Input: part model. Units: mm. Frame: model coordinates. Face numbers are marked on the shaded views. Give positions to 0.01 mm unless a question says otherwise; leave off trailing zeros. Write each loop counter-clockwise with the first axis right and the second up, starting at its lowest first coordinate (ties: lowest second). Pieces come first, ordered by that corner, then holes. Notation, with made-up numbers: (-6, 19) -> (3, 19) arc R27 cw to (3, 54) -> close; hole circle Ø8 at (12, 49.5). An arc over 180 degrees is marked (long way). Answer as a JSON object with one key per item and string values. Group by question number.
Autodesk Inventor part; units mm, degrees
ref_plane "YZ Plane" through (0, 0, 0) normal (1, 0, 0) x (0, 1, 0)
ref_plane "XZ Plane" through (0, 0, 0) normal (0, 1, 0) x (-1, 0, 0)
ref_plane "XY Plane" through (0, 0, 0) normal (0, 0, 1) x (1, 0, 0)
sketch "Sketch_1" plane through (0, 0, 0) normal (0, 0, 1) x (1, 0, 0)
  line L0 (12, 0) -> (-0.8, 0)
  line L1 (-0.8, 0) -> (-0.8, 2)
  line L2 (-0.8, 2) -> (-0.2226, 3)
  line L3 (-0.2226, 3) -> (0, 3)
  line L4 (0, 3) -> (0, 1.4467)
  arc A0 (0, 1.4467) -> (0.1, 1.3467) centre (0.1, 1.4467) ccw
  line L5 (0.1, 1.3467) -> (0.9, 1.3467)
  line L6 (0.9, 1.3467) -> (1.4, 1.5)
  line L7 (1.4, 1.5) -> (11.6935, 1.5)
  line L8 (11.6935, 1.5) -> (12, 1.1935)
  line L9 (12, 1.1935) -> (12, 0)
  line L10 (12, 0) -> (-0.8, 0)
revolve "Revolution1" add sketch "Sketch_1" angle 360 about axis through (12, 0, 0) along (1, 0, 0)
thread "Thread1"
sketch "Sketch2" plane through (-0.8, 0, 0) normal (-1, 0, 0) x (0, 0, 1)
  point P0 (0, 0)
hole "Hole1" at (-0.8, 0, 0) direction (1, 0, 0) diameter 1.5 depth 2 tip angle 120
sketch "Sketch_3" plane through (-0.8, 0, 0) normal (1, 0, 0) x (0, 0, -1)
  line L0 (-0.75, -0.433) -> (0, -0.866)
  line L1 (0, -0.866) -> (0.75, -0.433)
  line L2 (0.75, -0.433) -> (0.75, 0.433)
  line L3 (0.75, 0.433) -> (0, 0.866)
  line L4 (0, 0.866) -> (-0.75, 0.433)
  line L5 (-0.75, 0.433) -> (-0.75, -0.433)
extrude "Extrusion1" cut sketch "Sketch_3" along normal blind 2
properties part number "CBSTNR3-12" material "鋼、炭素鋼"
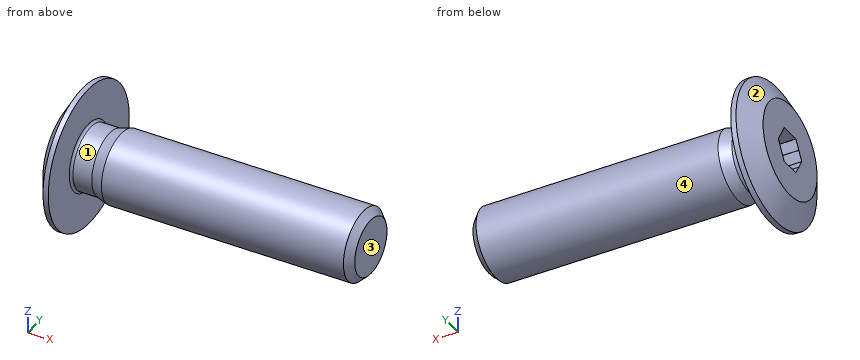
1. Line query: line 1 (Y direction, x = 6.5, z = -0.4); line 2 (X direction, y = 2.25, z = 0.1); line 3 (X direction, y = -0.25, z = 1.7). Output: solid intervals per line, ascending.
2. Contact query for flat-ended pins moving along their axis: pin 1 Ø3 at (x, z) = (5, 2.5) entering from +Y; pin 2 Ø2 at (x, y) = (8, 0) entering from -Z. Output: stop coordinate, or through.
3. Mould query, pull axis X, two halves, no side actions, for the marked faces 1, 2, 3 and 4. Classes: pulls with the +X half, pulls with the -X half, needs draft (parallel to the pull), parting line crosses it, or undercut.
4. Section B-B (x = 8). Return the cut outline in (y, z), plus the area to 3 significant figures.
Working result:
{
 "1": {"line 1": "y = -1.45 to 1.45", "line 2": "x = -0.65 to 0", "line 3": "x = -0.8 to 0"},
 "2": {"pin 1": "stops at y = 1.12", "pin 2": "stops at z = -1.5"},
 "3": {"face 1": "undercut", "face 2": "pulls with the -X half", "face 3": "pulls with the +X half", "face 4": "needs draft"},
 "4": {"outline": "circle Ø3 at (0, 0)", "area": "7.07 mm^2"}
}
